from build123d import *

# Parameters (mm, degrees)
PAD_DEPTH       = 8
SKETCH001_R     = 2
POCKET_DEPTH    = 9
SKETCH002_R     = 3.5
POCKET001_DEPTH = 5


with BuildPart() as part:
    # Sketch → Pad (new body)
    with BuildSketch(Plane.XY):
        with BuildLine():
            Line((0, 0), (0, 22.5))
            Line((0, 22.5), (4, 24.5))
            ThreePointArc((4, 22.5), (5, 23.5), (4, 24.5))
            Line((4, 22.5), (4, 11.5))
            Line((9, 11.5), (4, 11.5))
            Line((9, 0), (9, 11.5))
            Line((0, 0), (9, 0))
        make_face()
    extrude(amount=PAD_DEPTH)

    # Sketch001 (on Face6 of Pad) → Pocket (cut)
    with BuildSketch(Plane.YZ.offset(9)):
        with Locations((4.75, 4)):
            Circle(SKETCH001_R)
    extrude(amount=-POCKET_DEPTH, mode=Mode.SUBTRACT)

    # Sketch002 (on Face1 of Pocket) → Pocket001 (cut)
    with BuildSketch(Plane(origin=(0, 0, 0), x_dir=(0, -1, 0), z_dir=(-1, 0, 0))):
        with Locations((-4.75, 4)):
            Circle(SKETCH002_R)
    extrude(amount=-POCKET001_DEPTH, mode=Mode.SUBTRACT)


solid = part.part
The listing builds one solid part. Answer for the finished solid, in the listing's coordinates (mm). A direction names the side the tool comes from. Coordinates: 2 decimals unless noted, no trailing zeros. Write each loop counter-clockwise with the first axis right and the second up, starting at its lowest first coordinate (ties: lowest second). Pieces come first, ordered by that corner, then holes. Notation, with made-up numbers: (-18, 30.5) -> (15, 30.5) arc R34 ccw to (15, 67.5) -> close; hole circle Ø1 at (-12.5, 5). An arc over 180 degrees is marked (long way). One line per question, with ' | ' between items.
1. Section D-D (z = 5.25) is taken. Determine the outline of the cut face in (x, y).
Verdict:
outline: (0, 0) -> (9, 0) -> (9, 3.19) -> (5, 3.19) -> (5, 1.48) -> (0, 1.48) -> close; (0, 8.02) -> (5, 8.02) -> (5, 6.31) -> (9, 6.31) -> (9, 11.5) -> (4, 11.5) -> (4, 22.5) arc R1 ccw to (4, 24.5) -> (0, 22.5) -> close
2. Which of the six approach directions +Z, -Z, +X, -X, +Y, -Y give full straight-line access (tool end or side, diameter ignored) to faces 4 (the flat face through (0, 14, 4)), 5 (the flat face through (7, 11.5, 4)), 6 (the flat face through (5, 3, 2))?
Verdict:
face 4: +Z, -Z, -X, +Y, -Y | face 5: +Z, -Z, +X | face 6: -X
3. Given pin 1 Ø2.5 at (y, z) = (15.5, 4.5) entering from +X; pin 2 Ø3.5 at (y, z) = (6, 4.5) entering from -X; pin 3 Ø1.5 at (x, z) = (7.5, 7) entering from +Y, each flat-ended and moving along its own axis, determine where each tip first touches the part or whether it passes through.
Verdict:
pin 1: stops at x = 4 | pin 2: stops at x = 5 | pin 3: stops at y = 11.5
4. Section B-B (y = 4.75) is taken. Determine the outline of the cut face in (x, z).
Verdict:
outline: (0, 0) -> (9, 0) -> (9, 2) -> (5, 2) -> (5, 0.5) -> (0, 0.5) -> close; (0, 7.5) -> (5, 7.5) -> (5, 6) -> (9, 6) -> (9, 8) -> (0, 8) -> close
5. Section A-A (z = 4) is taken. Determine the outline of the cut face in (x, y).
Verdict:
outline: (0, 0) -> (9, 0) -> (9, 2.75) -> (5, 2.75) -> (5, 1.25) -> (0, 1.25) -> close; (0, 8.25) -> (5, 8.25) -> (5, 6.75) -> (9, 6.75) -> (9, 11.5) -> (4, 11.5) -> (4, 22.5) arc R1 ccw to (4, 24.5) -> (0, 22.5) -> close
6. For a pull along Y with two mould halves and no side action, classify faces 1 (the flat face through (4, 10, 8)), 2 (the flat face through (2, 23.5, 3.9)), 3 (the cylindrical face through (2.465, 3.135, 0.895)) as released by +Y, released by -Y, zero draft, split by the parting line, or undercut.
Verdict:
face 1: zero draft | face 2: released by +Y | face 3: undercut
7. Straight lines are drawn through the part: line 1 (Z direction, x = 6.65, y = 4.75); line 2 (Z direction, x = 3.05, y = 4.75); line 3 (Y direction, x = 4.75, z = 2.5). For each, find the intervals that lie inside material, in ascending order.
Verdict:
line 1: z = 0 to 2, 6 to 8 | line 2: z = 0 to 0.5, 7.5 to 8 | line 3: y = 0 to 1.59, 7.91 to 11.5, 22.84 to 24.16
8. Section C-C (x = 6) is taken. Determine the outline of the cut face in (y, z), and give its area (3 significant figures).
Verdict:
outline: (0, 0) -> (11.5, 0) -> (11.5, 8) -> (0, 8) -> close; hole circle Ø4 at (4.75, 4) | area: 79.4 mm^2
